Check sheet for the modelled part. Datum: model origin and axes. Units: mm. A direction names the side the tool comes from. Round coordinates to 2 decimals unless told otherwise and drop trailing zeros. Write each loop counter-clockwise with the first axis right and the second up, starting at its lowest first coordinate (ties: lowest second). Pieces come first, ordered by that corner, then holes. Notation, with made-up numbers: (-27, -18) - (4, -18) arc R7 cw to (4, -10) - close; hole circle Ø4 at (-32.75, 40). An arc over 180 degrees is marked (long way). Answer as a JSON object with one key per item and string values. Group by question number.
Item 1: Release check for a two-part mould opening along Z. For faces 3 (the flat face through (4, 0, 13)), 4 (the cylindrical face through (-0.195, 4.507, 3.513)), 5 (the flat face through (-4.5, 0.1, 26)) record: pulls with the +Z half, pulls with the -Z half, needs draft (parallel to the pull), parting line crosses it, or undercut.
Item 2: Sectioned sample at A-A on z = 21. Record the boundary of the cut face in (x, y).
Item 3: Sectioned sample at B-B on x = 3.5. Record the boundary of the cut face in (y, z).
Item 4: Sectioned sample at D-D on z = 15. Record the boundary of the cut face in (x, y), plus the area to 3 significant figures.
Item 5: Thickness scan on line 1 (X direction, y = -3.5, z = 16.25); line 2 (Z direction, x = 0, y = 4.45); line 3 (Y direction, x = -4.4, z = 15). Record the ranges inside material, lowest first.
Item 6: Sectioned sample at C-C on y = 0. Record the boundary of the cut face in (x, z), plus the area to 3 significant figures.
Item 7: Set-up check for faces 1 (the flat face through (0, -4, 13)), 2 (the cylindrical face through (-0.195, -4.493, 3.513)): record each of +Z, -Z, +X, -X, +Y, -Y from which the full face is reachable in a straight line by a thin tool's end or side.
```python
from build123d import *

# Parameters (mm, degrees)
SKETCH_1_W          = 10
SKETCH_1_H          = 10
SKETCH_1_W_2        = 8
SKETCH_1_H_2        = 8
EXTRUDE_1_DEPTH     = 26
SKETCH_2_R          = 1.5
CUT_EXTRUDE_1_DEPTH = 50
SKETCH_3_R          = 1.5
CUT_EXTRUDE_2_DEPTH = 10


with BuildPart() as part:
    # 草图1 → 拉伸-薄壁1 (new body)
    with BuildSketch(Plane.XY):
        Rectangle(SKETCH_1_W, SKETCH_1_H)
        Rectangle(SKETCH_1_W_2, SKETCH_1_H_2, mode=Mode.SUBTRACT)
    extrude(amount=EXTRUDE_1_DEPTH)

    # 草图2 → 切除-拉伸1 (cut)
    with BuildSketch(Plane(origin=(0, 5, 0), x_dir=(1, 0, 0), z_dir=(0, 1, 0))):
        with Locations((0, -5)):
            Circle(SKETCH_2_R)
    extrude(amount=-CUT_EXTRUDE_1_DEPTH, mode=Mode.SUBTRACT)

    # 草图3 → 切除-拉伸2 (cut)
    with BuildSketch(Plane(origin=(5, 0, 0), x_dir=(0, 0, -1), z_dir=(1, 0, 0))):
        with Locations((-15, 0)):
            Circle(SKETCH_3_R)
    extrude(amount=-CUT_EXTRUDE_2_DEPTH, mode=Mode.SUBTRACT)


solid = part.part
```
Completed:
{
 "1": {"face 3": "needs draft", "face 4": "undercut", "face 5": "pulls with the +Z half"},
 "2": {"outline": "(-5, -5) - (5, -5) - (5, 5) - (-5, 5) - close; hole (-4, -4) - (4, -4) - (4, 4) - (-4, 4) - close"},
 "3": {"outline": "(-5, 0) - (-4, 0) - (-4, 26) - (-5, 26) - close; (4, 0) - (5, 0) - (5, 26) - (4, 26) - close"},
 "4": {"outline": "(-5, -5) - (5, -5) - (5, -1.5) - (4, -1.5) - (4, -4) - (-4, -4) - (-4, -1.5) - (-5, -1.5) - close; (-5, 1.5) - (-4, 1.5) - (-4, 4) - (4, 4) - (4, 1.5) - (5, 1.5) - (5, 5) - (-5, 5) - close", "area": "30.0 mm²"},
 "5": {"line 1": "-5 to -4, 4 to 5", "line 2": "0 to 3.5, 6.5 to 26", "line 3": "-5 to -1.5, 1.5 to 5"},
 "6": {"outline": "(-5, 0) - (-4, 0) - (-4, 13.5) - (-5, 13.5) - close; (-5, 16.5) - (-4, 16.5) - (-4, 26) - (-5, 26) - close; (4, 0) - (5, 0) - (5, 13.5) - (4, 13.5) - close; (4, 16.5) - (5, 16.5) - (5, 26) - (4, 26) - close", "area": "46.0 mm²"},
 "7": {"face 1": "+Z, -Z", "face 2": "+Y, -Y"}
}
